Could you check a few things on this model? Use its own coordinates, in mm. Face numbers are marked on the shaded views. A direction names the side the tool comes from. Coordinates: 2 decimals unless noted, no trailing zeros. Loops run counter-clockwise (first coordinate to the right, second up) from the corner with the lowest first, then second, coordinate; pieces in that order, holes last.
Autodesk Inventor part; units mm, degrees
ref_plane "YZ Plane" through (0, 0, 0) normal (1, 0, 0) x (0, 1, 0)
ref_plane "XZ Plane" through (0, 0, 0) normal (0, 1, 0) x (-1, 0, 0)
ref_plane "XY Plane" through (0, 0, 0) normal (0, 0, 1) x (1, 0, 0)
sketch "Sketch1" plane through (0, 0, 0) normal (0, 0, 1) x (1, 0, 0)
  arc A0 (8.9398, 3.175) -> (8.9398, -3.175) centre (0, 0) ccw
  arc A1 (9.0696, 8.89) -> (9.0696, -8.89) centre (0, 0) ccw
  line L0 (8.9398, 3.175) -> (12.2967, 3.175)
  line L1 (8.9398, -3.175) -> (12.2967, -3.175)
  line L2 (12.2967, 3.175) -> (22.4567, 3.175)
  line L3 (12.2967, -3.175) -> (22.4567, -3.175)
  line L4 (22.4567, 3.175) -> (22.4567, 6.985)
  line L5 (22.4567, 6.985) -> (13.6044, 6.985)
  line L6 (22.4567, -3.175) -> (22.4567, -6.985)
  line L7 (22.4567, -6.985) -> (13.6044, -6.985)
  line L8 (-18.034, 0) -> (28.275, 0) construction
  arc A2 (9.0696, 8.89) -> (13.6044, 6.985) centre (13.6044, 13.335) ccw
  arc A3 (13.6044, -6.985) -> (9.0696, -8.89) centre (13.6044, -13.335) ccw
  point P0 (10.6066, 6.985)
  point P1 (10.6066, -6.985)
  dimension "d0" = 18.9738
  dimension "d1" = 25.4
  dimension "d8" = 3.81
  dimension "d18" = 3.175
  dimension "d19" = 6.35
  dimension "d20" = 13.5169
  dimension "d21" = 8.8523
extrude "Extrusion1" add sketch "Sketch1" along normal blind 6.35
sketch "Sketch2" plane through (13.6044, 6.985, 0) normal (0, 1, 0) x (1, 0, 0)
  line L0 (0, 0) -> (8.8523, 0)
  line L1 (8.8523, -6.35) -> (0, -6.35)
  line L2 (4.4262, -6.35) -> (4.4262, 0) construction
  point P0 (-13.6044, 0)
  point P1 (4.4262, -3.175)
hole "Hole1" at (18.0306, 6.985, 3.175) direction (0, -1, 0) diameter 3.6576 end up to surface
sketch "Sketch3" plane through (13.6044, -6.985, 0) normal (0, -1, 0) x (1, 0, 0)
  circle A0 centre (4.4262, 3.175) radius 1.8288
  point P0 (-13.6044, 0)
hole "Hole2" at (18.0306, -6.985, 3.175) direction (0, 1, 0) diameter 3.302 end up to surface
properties part number "bearing_blcok"
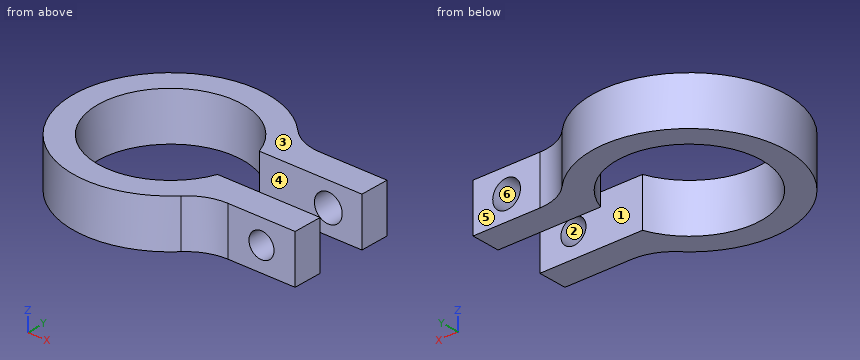
1) Imagine slicing it at B-B on x = 12. List the corners of the cut face in (y, z) for me (3 decimals), plus the area to 3 significant figures.
2) Imagine slicing it at D-D on x = 0. List the corners of the cut face in (y, z) for me.
3) Will these pins go through, and if not, where does the flat tip stop? pin 1 (3 mm diameter, centred on x = 17.5, z = 4, fed in from +Y) (3 decimals); pin 2 (3 mm diameter, centred on x = 17, z = 3, fed in from -Y) (3 decimals).
4) Imagine slicing it at C-C on z = 3.25. List the corners of the cut face in (x, y) for me (3 decimals), plus the area to 3 significant figures.
5) If I drill on L1, parallel to Y at x = 14, z = 0.5 (3 decimals); L2, parallel to X at y = -3.5, z = 3.75; L3, parallel to X at y = 5.75, z = 3.25, over which ranges is the centre line in solid material (lowest first)?
6) For the marked faces 4, 5 and 6, which set-ups out of +Z, -Z, +X, -X, +Y, -Y let a thin tool reach every point of the face, with its end or its side?
7) Imagine slicing it at A-A on y = -6. List the corners of the cut face in (x, z) for me (3 decimals), plus the area to 3 significant figures.
8) We'd pull the mould along Z, two halves only. Please class the marked faces 1, 2 and 3: released by +Z, released by -Z, zero draft, split by the parting line, or undercut.
Solved:
1. outline: (-7.191, 0) - (-3.175, 0) - (-3.175, 6.35) - (-7.191, 6.35) - close; (3.175, 0) - (7.191, 0) - (7.191, 6.35) - (3.175, 6.35) - close
1. area: 51.0 mm2
2. outline: (-12.7, 0) - (-9.49, 0) - (-9.49, 6.35) - (-12.7, 6.35) - close; (9.49, 0) - (12.7, 0) - (12.7, 6.35) - (9.49, 6.35) - close
3. pin 1: stops at y = 6.985
3. pin 2: stops at y = -6.985
4. outline: (8.94, -3.175) arc R9.487 cw (long way) to (8.94, 3.175) - (16.203, 3.175) - (16.203, 6.985) - (13.604, 6.985) arc R6.35 cw to (9.07, 8.89) arc R12.7 ccw (long way) to (9.07, -8.89) arc R6.35 cw to (13.604, -6.985) - (16.381, -6.985) - (16.381, -3.175) - close; (19.68, -6.985) - (22.457, -6.985) - (22.457, -3.175) - (19.68, -3.175) - close; (19.858, 3.175) - (22.457, 3.175) - (22.457, 6.985) - (19.858, 6.985) - close
4. area: 262 mm2
5. L1: y = -6.985 to -3.175, 3.175 to 6.985
5. L2: x = -12.21 to -8.82, 8.82 to 16.48, 19.58 to 22.46
5. L3: x = -11.32 to -7.55, 7.55 to 16.2, 19.86 to 22.46
6. face 4: +Z, -Z, +X
6. face 5: +Z, -Z, +X, +Y
6. face 6: +Y
7. outline: (-11.193, 0) - (-7.349, 0) - (-7.349, 6.35) - (-11.193, 6.35) - close; (7.349, 0) - (22.457, 0) - (22.457, 6.35) - (7.349, 6.35) - close; hole circle Ø3.302 at (18.031, 3.175)
7. area: 112 mm2
8. face 1: zero draft
8. face 2: undercut
8. face 3: released by +Z
